Check sheet for the drawn part. Datum: minimum x, y, z corner. Units: mm. Coordinates: 2 decimals unless noted, no trailing zeros. Write each loop counter-clockwise with the first axis right and the second up, starting at its lowest first coordinate (ties: lowest second). Pieces come first, ordered by that corner, then holes. Notation, with made-up numbers: (33, 85.5) - (67, 85.5) arc R30 cw to (67, 108.5) - close; hole circle Ø3 at (-13, 61). An arc over 180 degrees is marked (long way). Use one line per item in the form item = value. Start each with the question number.
1. Cross-section at A-A on x = 3.45. Record the boundary of the cut face in (y, z), then the cut area to 3 significant figures.
2. Scan lines: line 1 along Y through (x, z) = (3.55, 0.95); line 2 along Z through (x, y) = (3.2, 11.25); line 3 along Y through (x, z) = (2.45, 3.1). Record each from-to range of solid material in increasing order.
3. Cross-section at B-B on z = 1.95. Record the boundary of the cut face in (x, y), then the cut area to 3 significant figures.
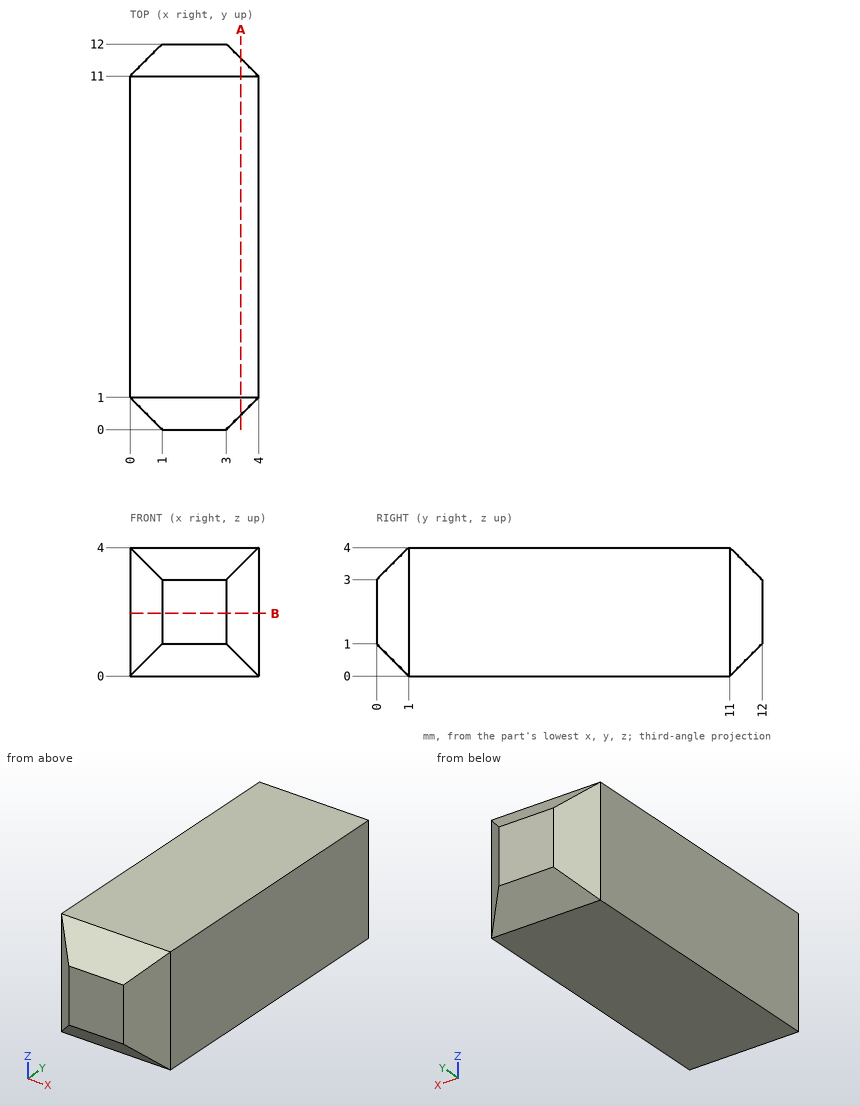
Final values:
q1.outline = (0.45, 0.55) - (1, 0) - (11, 0) - (11.55, 0.55) - (11.55, 3.45) - (11, 4) - (1, 4) - (0.45, 3.45) - close
q1.area = 43.8 mm²
q2.line_1 = 0.55 to 11.45
q2.line_2 = 0.25 to 3.75
q2.line_3 = 0.1 to 11.9
q3.outline = (0, 1) - (1, 0) - (3, 0) - (4, 1) - (4, 11) - (3, 12) - (1, 12) - (0, 11) - close
q3.area = 46.0 mm²
